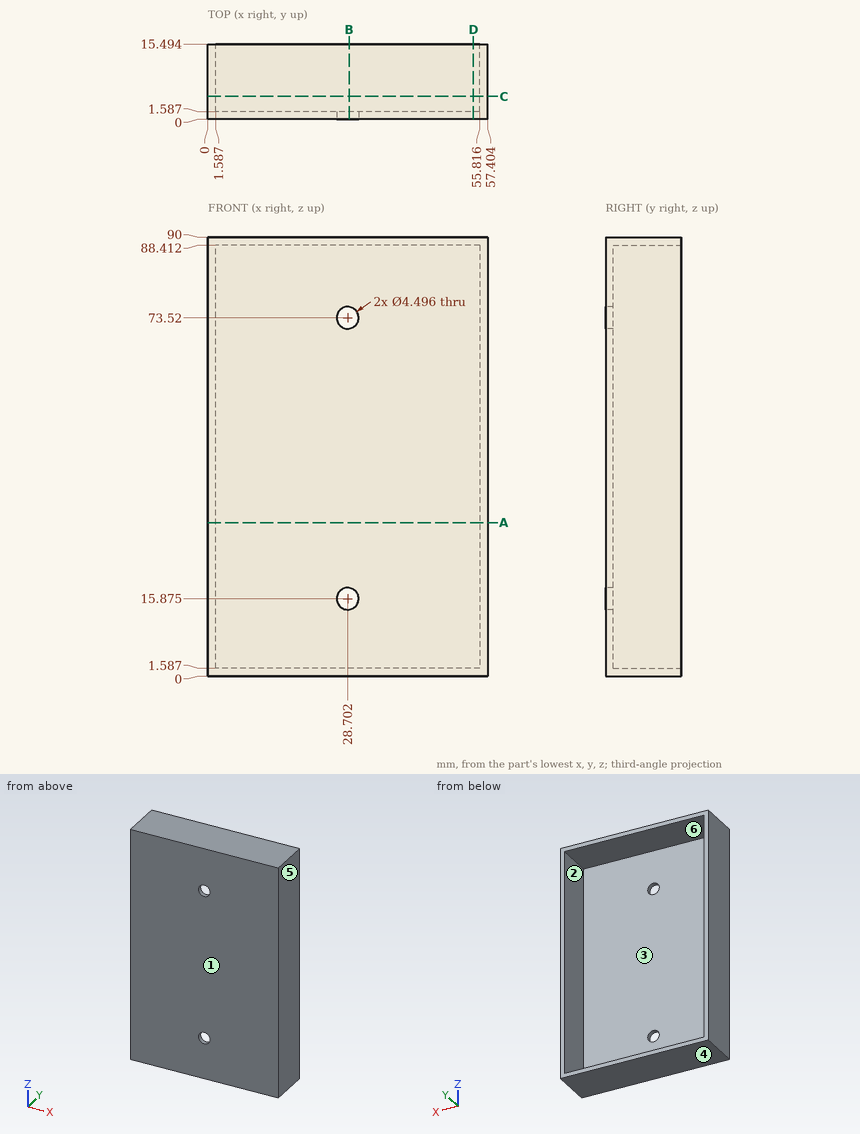
The drawing under review shows one solid part. Ordinate dimensions are in mm from its lowest x, y, z. A direction names the side the tool comes from. Round coordinates to 2 decimals unless told otherwise and drop trailing zeros. Write each loop counter-clockwise with the first axis right and the second up, starting at its lowest first coordinate (ties: lowest second). Pieces come first, ordered by that corner, then holes. Notation, with made-up numbers: (-10, -9.75) - (27, -9.75) arc R19 cw to (27, 5.25) - close; hole circle Ø2 at (5.25, 87). An arc over 180 degrees is marked (long way). Put each result on its own line as item: value.
Q1. We need section A-A (z = 31.5). Give the boundary of the cut face in (x, y) (1 decimal), and give its area (3 significant figures).
Solved:
outline: (0, 0) - (57.4, 0) - (57.4, 15.5) - (55.8, 15.5) - (55.8, 1.6) - (1.6, 1.6) - (1.6, 15.5) - (0, 15.5) - close
area: 135 mm2
Q2. We need section C-C (y = 4.75). Give the boundary of the cut face in (x, z) (1 decimal).
Solved:
outline: (0, 0) - (57.4, 0) - (57.4, 90) - (0, 90) - close; hole (1.6, 1.6) - (55.8, 1.6) - (55.8, 88.4) - (1.6, 88.4) - close
Q3. We need section D-D (x = 54.5). Give the boundary of the cut face in (y, z) (1 decimal).
Solved:
outline: (0, 0) - (15.5, 0) - (15.5, 1.6) - (1.6, 1.6) - (1.6, 88.4) - (15.5, 88.4) - (15.5, 90) - (0, 90) - close
Q4. We need section B-B (x = 29). Give the boundary of the cut face in (y, z) (1 decimal), and give its area (3 significant figures).
Solved:
outline: (0, 0) - (15.5, 0) - (15.5, 1.6) - (1.6, 1.6) - (1.6, 13.6) - (0, 13.6) - close; (0, 18.1) - (1.6, 18.1) - (1.6, 71.3) - (0, 71.3) - close; (0, 75.7) - (1.6, 75.7) - (1.6, 88.4) - (15.5, 88.4) - (15.5, 90) - (0, 90) - close
area: 173 mm2
Q5. Insertion check: pin 1 Ø16.5 at (x, z) = (33.5, 34) entering from +Y. The pin has a flat end and moves straight along its axis. Give the tip position at first contact, or say it passes through.
Solved:
pin 1: stops at y = 1.59
Q6. Mouldability with a two-part tool opening along Z and no side actions: class the marked faces 1, 2, 3 and 4 as released by +Z, released by -Z, zero draft, split by the parting line, or undercut.
Solved:
face 1: zero draft
face 2: undercut
face 3: undercut
face 4: released by -Z
Q7. Wall thickness on probe 1 along Z at (x, y) = (39, 11.75); probe 2 along X at (y, z) = (8, 16.5) (1 decimal); probe 3 along Y at (x, z) = (10, 68): over which ranges is each line inside the solid? List them lowest first.
Solved:
probe 1: z = 0 to 1.59, 88.41 to 90
probe 2: x = 0 to 1.6, 55.8 to 57.4
probe 3: y = 0 to 1.59
Q8. Machinability: for the marked faces 5 and 6, which of the approach directions +Z, -Z, +X, -X, +Y, -Y give a long, thin tool a straight path to every point of the face, cutting with its end or side? Answer none if there is none.
Solved:
face 5: +Z, -Z, +X, +Y, -Y
face 6: +Y
